Input: part model. Units: mm. Frame: model coordinates. A direction names the side the tool comes from. Coordinates: 2 decimals unless noted, no trailing zeros. Write each loop counter-clockwise with the first axis right and the second up, starting at its lowest first coordinate (ties: lowest second). Pieces come first, ordered by that corner, then holes. Notation, with made-up numbers: M 48,8.5 L 75,8.5 A31 cw 75,44.5 Z; hole C -26.5,-28.5 d11. An arc over 180 degrees is marked long. Answer as a JSON object with one key per item and string values. Group by question number.
from build123d import *

# Parameters (mm, degrees)
BOSS_EXTRUDE1_DEPTH = 17
SKETCH2_W           = 44
SKETCH2_H           = 17
BOSS_EXTRUDE2_DEPTH = 2.15
SKETCH3_R           = 6.275
BOSS_EXTRUDE3_DEPTH = 3
SKETCH4_R           = 1.5
BOSS_EXTRUDE4_DEPTH = 3


with BuildPart() as part:
    # Sketch1 → Boss-Extrude1 (new body)
    with BuildSketch(Plane.XY):
        Polygon((-16, 12.5), (-6, 15.5), (16, 15.5), (16, -15.5), (-16, -15.5), align=None)
    extrude(amount=-BOSS_EXTRUDE1_DEPTH)

    # Sketch2 → Boss-Extrude2 (add)
    with BuildSketch(Plane(origin=(0, 7.5, 0), x_dir=(1, 0, 0), z_dir=(0, 1, 0))):
        with Locations((0, 8.5)):
            Rectangle(SKETCH2_W, SKETCH2_H)
    extrude(amount=BOSS_EXTRUDE2_DEPTH)

    # Sketch3 → Boss-Extrude3 (add)
    with BuildSketch(Plane(origin=(0, 15.5, 0), x_dir=(1, 0, 0), z_dir=(0, 1, 0))):
        with Locations(Location((7, 8.5, 0), (0, 0, 180))):
            Circle(SKETCH3_R)
    extrude(amount=BOSS_EXTRUDE3_DEPTH)

    # Sketch4 → Boss-Extrude4 (add)
    with BuildSketch(Plane(origin=(0, 18.5, 0), x_dir=(1, 0, 0), z_dir=(0, 1, 0))):
        with Locations(Location((7, 8.5, 0), (0, 0, 180))):
            Circle(SKETCH4_R)
    extrude(amount=BOSS_EXTRUDE4_DEPTH)


solid = part.part
Q1. Pin query (flat end, axial travel): pin 1 Ø5 at (y, z) = (1, -8.5) entering from -X; pin 2 Ø1.8 at (y, z) = (12.5, -5.5) entering from +X; pin 3 Ø1.8 at (x, z) = (-20, -11) entering from -Y. Return the tip coordinate at first contact, or that it passes through.
Q2. Section B-B, the plane z = -8.5. Return the cut outline in (x, y) (3 decimals), and give its area (3 significant figures).
Q3. Section D-D, the plane z = -0.75. Return the cut outline in (x, y), and give its area (3 significant figures).
Q4. Access query for faces 1 (the flat face through (19, 9.65, -9)), 2 (the flat face through (-16, -4, -8)), 3 (the flat face through (-16, 11, -8)). Directions: +Z, -Z, +X, -X, +Y, -Y. A direction counts if a zero-diameter tool reaches every point of the face in a straight line with its end or side. Return the directions, or none.
Q5. Section C-C, the plane y = 18. Return the cut outline in (x, z) (3 decimals), and give its area (3 significant figures).
Q6. Line query: line 1 (Y direction, x = 15.5, z = -2); line 2 (X direction, y = 11, z = -4.5); line 3 (Y direction, x = 16.5, z = -15). Output: solid intervals per line, ascending. Write a range as from..to.
Q7. Section A-A, the plane x = 7. Return the cut outline in (y, z) (3 decimals), and give its area (3 significant figures).
Filled in:
{
 "1": {"pin 1": "x = -16", "pin 2": "x = 16", "pin 3": "y = 7.5"},
 "2": {"outline": "M -22,7.5 L -16,7.5 L -16,-15.5 L 16,-15.5 L 16,7.5 L 22,7.5 L 22,9.65 L 16,9.65 L 16,15.5 L 13.275,15.5 L 13.275,18.5 L 8.5,18.5 L 8.5,21.5 L 5.5,21.5 L 5.5,18.5 L 0.725,18.5 L 0.725,15.5 L -6,15.5 L -16,12.5 L -16,9.65 L -22,9.65 Z", "area": "1,050 mm^2"},
 "3": {"outline": "M -22,7.5 L -16,7.5 L -16,-15.5 L 16,-15.5 L 16,7.5 L 22,7.5 L 22,9.65 L 16,9.65 L 16,15.5 L -6,15.5 L -16,12.5 L -16,9.65 L -22,9.65 Z", "area": "1,000 mm^2"},
 "4": {"face 1": "+Z, -Z, +X, +Y", "face 2": "+Z, -Z, -X, -Y", "face 3": "+Z, -Z, -X, +Y"},
 "5": {"outline": "C 7,-8.5 d12.55", "area": "124 mm^2"},
 "6": {"line 1": "-15.5..15.5", "line 2": "-16..16", "line 3": "7.5..9.65"},
 "7": {"outline": "M -15.5,-17 L 15.5,-17 L 15.5,-14.775 L 18.5,-14.775 L 18.5,-10 L 21.5,-10 L 21.5,-7 L 18.5,-7 L 18.5,-2.225 L 15.5,-2.225 L 15.5,0 L -15.5,0 Z", "area": "574 mm^2"}
}
